from build123d import *

# Parameters (mm, degrees)
F0_W        = 50.292
F0_H        = 25.908
F1_DEPTH    = 10.16
F2_W        = 47.752
F2_H        = 23.368
F3_DEPTH    = 8.89
F4_T1_DEPTH = 19.3581536726
F4_T3_DEPTH = 35.1061536726
F5_T1_DEPTH = 19.3581536726
F5_T3_DEPTH = 35.1061536726


# Not quite as in the source:
# - a fillet or chamfer that OpenCascade refuses, or shapes differently, is made with other operations: its cross-section is extruded or revolved along the edge and cut away or added
# - a feature names something its author has since deleted; it is built from what else it names


with BuildPart() as f1:
    # F0 (on Top) → F1 (new body)
    with BuildSketch(Plane.XY):
        Rectangle(F0_W, F0_H)
    extrude(amount=F1_DEPTH)

    # F2 (on face) → F3 (cut)
    with BuildSketch(Plane.XY.offset(10.16)):
        Rectangle(F2_W, F2_H)
    extrude(amount=-F3_DEPTH, mode=Mode.SUBTRACT)

    # F4: fillet of radius 1.8396307345 on 4 edges, made by hand

    # F4_s2 → F4_t1 (cut)
    with BuildSketch(Plane.XY.offset(-4.5990768363)):
        with BuildLine():
            ThreePointArc((-23.3063692655, 12.954), (-24.6071846327, 12.4151846327), (-25.146, 11.1143692655))
            Line((-25.146, 11.1143692655), (-25.146, 12.954))
            Line((-25.146, 12.954), (-23.3063692655, 12.954))
        make_face()
        with BuildLine():
            ThreePointArc((-25.146, -11.1143692655), (-24.6071846327, -12.4151846327), (-23.3063692655, -12.954))
            Line((-23.3063692655, -12.954), (-25.146, -12.954))
            Line((-25.146, -12.954), (-25.146, -11.1143692655))
        make_face()
    extrude(amount=F4_T1_DEPTH, mode=Mode.SUBTRACT)

    # F4_s4 → F4_t3 (cut)
    with BuildSketch(Plane.XZ.offset(-17.5530768363)):
        with BuildLine():
            ThreePointArc((-25.146, 1.8396307345), (-24.6071846327, 0.5388153673), (-23.3063692655, 0))
            Line((-23.3063692655, 0), (-25.146, 0))
            Line((-25.146, 0), (-25.146, 1.8396307345))
        make_face()
        with BuildLine():
            ThreePointArc((-25.146, 8.3203692655), (-24.6071846327, 9.6211846327), (-23.3063692655, 10.16))
            Line((-23.3063692655, 10.16), (-25.146, 10.16))
            Line((-25.146, 10.16), (-25.146, 8.3203692655))
        make_face()
    extrude(amount=F4_T3_DEPTH, mode=Mode.SUBTRACT)

    # F5: fillet of radius 1.8396307345 on 4 edges, made by hand

    # F5_s2 → F5_t1 (cut)
    with BuildSketch(Plane.XY.offset(-4.5990768363)):
        with BuildLine():
            ThreePointArc((25.146, -11.1143692655), (24.6071846327, -12.4151846327), (23.3063692655, -12.954))
            Line((23.3063692655, -12.954), (25.146, -12.954))
            Line((25.146, -12.954), (25.146, -11.1143692655))
        make_face()
        with BuildLine():
            ThreePointArc((23.3063692655, 12.954), (24.6071846327, 12.4151846327), (25.146, 11.1143692655))
            Line((25.146, 11.1143692655), (25.146, 12.954))
            Line((25.146, 12.954), (23.3063692655, 12.954))
        make_face()
    extrude(amount=F5_T1_DEPTH, mode=Mode.SUBTRACT)

    # F5_s4 → F5_t3 (cut)
    with BuildSketch(Plane.XZ.offset(-17.5530768363)):
        with BuildLine():
            ThreePointArc((23.3063692655, 0), (24.6071846327, 0.5388153673), (25.146, 1.8396307345))
            Line((25.146, 1.8396307345), (25.146, 0))
            Line((25.146, 0), (23.3063692655, 0))
        make_face()
        with BuildLine():
            ThreePointArc((23.3063692655, 10.16), (24.6071846327, 9.6211846327), (25.146, 8.3203692655))
            Line((25.146, 8.3203692655), (25.146, 10.16))
            Line((25.146, 10.16), (23.3063692655, 10.16))
        make_face()
    extrude(amount=F5_T3_DEPTH, mode=Mode.SUBTRACT)


solid = f1.part
Verification items for the finished model (mm, model axes). A direction names the side the tool comes from. Round coordinates to 2 decimals unless told otherwise and drop trailing zeros. Order: outer loops, then holes, each group sorted by start corner. A loop starts at its lowest first (then second) coordinate and runs counter-clockwise, first axis right, second up. Notation, with made-up numbers: (52, 77.25) -> (96, 77.25) arc R15 cw to (96, 100.25) -> close; hole circle Ø9 at (47, 28.25). An arc over 180 degrees is marked (long way). Put each result on its own line as item: value.
1) Material ranges on line 1 (X direction, y = 2.75, z = 7); line 2 (Y direction, x = -5, z = 3.75); line 3 (Z direction, x = 20, y = 8.75), recorded low to high.
Final values:
line 1: x = -25.15 to -23.88, 23.88 to 25.15
line 2: y = -12.95 to -11.68, 11.68 to 12.95
line 3: z = 0 to 1.27
2) Section check A-A (z = 4.25). Record the cut outline in (x, y), then the cut area to 3 significant figures.
Final values:
outline: (-25.15, -11.11) arc R1.84 ccw to (-23.31, -12.95) -> (23.31, -12.95) arc R1.84 ccw to (25.15, -11.11) -> (25.15, 11.11) arc R1.84 ccw to (23.31, 12.95) -> (-23.31, 12.95) arc R1.84 ccw to (-25.15, 11.11) -> close; hole (-23.88, -11.68) -> (23.88, -11.68) -> (23.88, 11.68) -> (-23.88, 11.68) -> close
area: 184 mm^2
3) Set-up check for faces 4 (the flat face through (0, -11.684, 6)), 5 (the cylindrical face through (-24.825, 0.181, 9.359)): record each of +Z, -Z, +X, -X, +Y, -Y from which the full face is reachable in a straight line by a thin tool's end or side.
Final values:
face 4: +Z
face 5: +Z, -X, +Y, -Y
4) Mould release check, pull along Y, two halves, no side actions. Record for faces 1 (the flat face through (-23.876, 0, 6)), 2 (the cylindrical face through (-24.62, -12.4, 5.01)), 3 (the cylindrical face through (24.59, 0.18, 0.52)): +Y half, -Y half, draft (parallel to the pull), parting line (faces both ways), or undercut.
Final values:
face 1: undercut
face 2: -Y half
face 3: draft
5) Section check B-B (x = -10.5). Record the cut outline in (y, z), then the cut area to 3 significant figures.
Final values:
outline: (-12.95, 0) -> (12.95, 0) -> (12.95, 10.16) -> (11.68, 10.16) -> (11.68, 1.27) -> (-11.68, 1.27) -> (-11.68, 10.16) -> (-12.95, 10.16) -> close
area: 55.5 mm^2
6) Section check C-C (y = -10.5). Record the cut outline in (x, z), then the cut area to 3 significant figures.
Final values:
outline: (-25.15, 1.84) arc R1.84 ccw to (-23.31, 0) -> (23.31, 0) arc R1.84 ccw to (25.15, 1.84) -> (25.15, 8.32) arc R1.84 ccw to (23.88, 10.07) -> (23.88, 1.27) -> (-23.88, 1.27) -> (-23.88, 10.07) arc R1.84 ccw to (-25.15, 8.32) -> close
area: 83.6 mm^2
